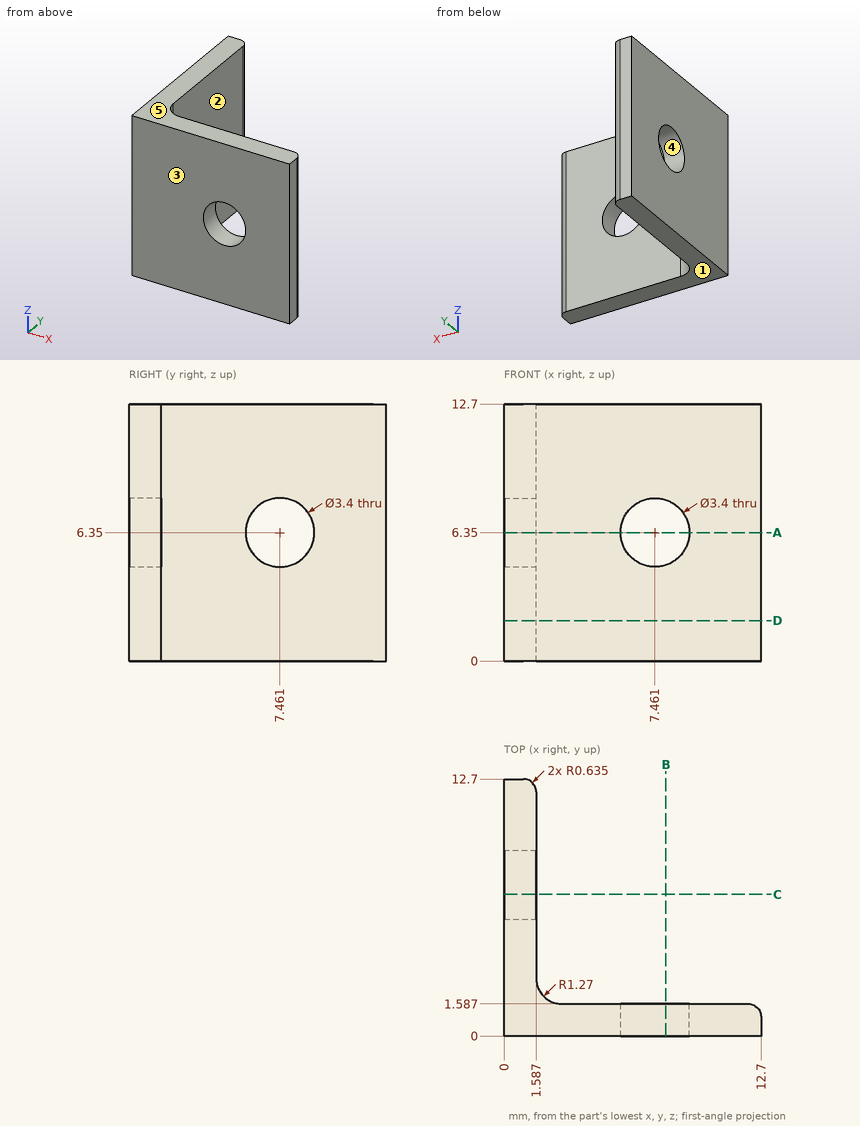
Drawing for the job (mm, zero at the part's lowest x, y, z). A direction names the side the tool comes from. Give positions to 0.01 mm unless a question says otherwise; leave off trailing zeros. Order: outer loops, then holes, each group sorted by start corner. A loop starts at its lowest first (then second) coordinate and runs counter-clockwise, first axis right, second up. Notation, with made-up numbers: (80, 36) - (114, 36) arc R21 ccw to (114, 66) - close; hole circle Ø10 at (13.25, -13). An arc over 180 degrees is marked (long way). Write item = value, one per line. Start each with the question number.
1. Drop flat-ended pins along their axis: P1, Ø2, axis at y = 7.46, z = 6.35, coming from the -X side; P2, Ø4, axis at x = 4.5, z = 2.5, coming from the +Y side; P3, Ø7.5, axis at y = 6, z = 8.5, coming from the +X side. Give the stop position or say it passes through.
2. Two-plate mould, pull along Z, no slides. Class the marked faces 3, 4 and 5: pulls with the +Z half, pulls with the -Z half, needs draft (parallel to the pull), parting line crosses it, or undercut.
3. Which spindle directions (+Z, -Z, +X, -X, +Y, -Y) get a long thin tool onto all of the face, cutting with end or side? Do the marked faces 1 and 2. Say none if no direction does.
4. Cut at B-B, the plane x = 8. List the corners of the cut face in (y, z).
5. Cut at D-D, the plane z = 2. List the corners of the cut face in (x, y) (1 decimal).
6. Cut at C-C, the plane y = 7. List the corners of the cut face in (x, z).
7. Cut at A-A, the plane z = 6.35. List the corners of the cut face in (x, y) (1 decimal).
8. Probe line 1 along X through (y, z) = (0.55, 6.35); line 2 along Y through (x, z) = (3, 7). List the from-to ranges inside material, lowest first.
Taken from the geometry:
q1.P1 = through
q1.P2 = 1.64
q1.P3 = 1.74
q2.face_3 = needs draft
q2.face_4 = undercut
q2.face_5 = pulls with the +Z half
q3.face_1 = -Z, +X, -X, +Y, -Y
q3.face_2 = +Z, -Z, +X, +Y
q4.outline = (0, 0) - (1.59, 0) - (1.59, 4.74) - (0, 4.74) - close; (0, 7.96) - (1.59, 7.96) - (1.59, 12.7) - (0, 12.7) - close
q5.outline = (0, 0) - (12.7, 0) - (12.7, 1) arc R0.6 ccw to (12.1, 1.6) - (2.9, 1.6) arc R1.3 cw to (1.6, 2.9) - (1.6, 12.1) arc R0.6 ccw to (1, 12.7) - (0, 12.7) - close
q6.outline = (0, 0) - (1.59, 0) - (1.59, 4.71) - (0, 4.71) - close; (0, 7.99) - (1.59, 7.99) - (1.59, 12.7) - (0, 12.7) - close
q7.outline = (0, 0) - (5.8, 0) - (5.8, 1.6) - (2.9, 1.6) arc R1.3 cw to (1.6, 2.9) - (1.6, 5.8) - (0, 5.8) - close; (0, 9.2) - (1.6, 9.2) - (1.6, 12.1) arc R0.6 ccw to (1, 12.7) - (0, 12.7) - close; (9.2, 0) - (12.7, 0) - (12.7, 1) arc R0.6 ccw to (12.1, 1.6) - (9.2, 1.6) - close
q8.line_1 = 0 to 5.76, 9.16 to 12.7
q8.line_2 = 0 to 1.59
